Build history of the part. All positions in model axes, mm. Round coordinates to 2 decimals unless told otherwise and drop trailing zeros. Loops run counter-clockwise (first coordinate to the right, second up) from the corner with the lowest first, then second, coordinate; pieces in that order, holes last. Notation, with made-up numbers: M 74.25,68 L 125.25,68 A19 cw 125.25,100 Z; hole C 53.5,61.25 d1. An arc over 180 degrees is marked long. Use one line per item in the form item = value. Start each with the question number.
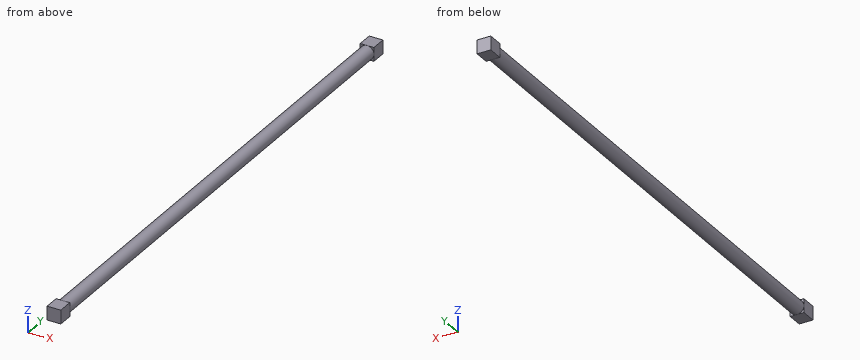
```python
from build123d import *

# Parameters (mm, degrees)
F0_R     = 5.715
F1_DEPTH = 457.2
F2_W     = 11.43
F2_H     = 11.43
F3_DEPTH = 12.7
F4_W     = 11.43
F4_H     = 11.43
F5_DEPTH = 12.7


with BuildPart() as f1:
    # F0 (on Front) → F1 (new body)
    with BuildSketch(Plane.XZ):
        Circle(F0_R)
    extrude(amount=F1_DEPTH)

    # F2 (on face) → F3 (join)
    with BuildSketch(Plane(origin=(0, 0, 0), x_dir=(-1, 0, 0), z_dir=(0, 1, 0))):
        Rectangle(F2_W, F2_H)
    extrude(amount=-F3_DEPTH)

    # F4 (on face) → F5 (join)
    with BuildSketch(Plane.XZ.offset(457.2)):
        Rectangle(F4_W, F4_H)
    extrude(amount=-F5_DEPTH)


solid = f1.part
```
Q1. Wall check: probe 1 along Y at (x, z) = (5.25, -5); probe 2 along Z at (x, y) = (0.25, -436.5); probe 3 along Z at (x, y) = (1, -319). Give the ranges that are in metal, low to high.
Q2. Saw through at C-C (y = -225). Give the cut face in (x, z) (3 decimals).
Q3. Saw through at B-B (z = 1.75). Give the cut face in (x, y) (3 decimals).
Q4. Drop flat-ended pins along their axis: P1, Ø4.5, axis at x = -3.5, z = 3.5, coming from the +Y side; P2, Ø2, axis at y = -92, z = -2, coming from the -X side; P3, Ø2, axis at x = -4, y = -174.5, coming from the +Z side. Give the stop position or say it passes through.
Q5. Saw through at A-A (x = -2.5). Give the cut face in (y, z) (3 decimals), and give its area (3 significant figures).
Filled in:
q1.probe_1 = -457.2 to -444.5, -12.7 to 0
q1.probe_2 = -5.71 to 5.71
q1.probe_3 = -5.63 to 5.63
q2.outline = C 0,0 d11.43
q3.outline = M -5.715,-457.2 L 5.715,-457.2 L 5.715,-444.5 L 5.44,-444.5 L 5.44,-12.7 L 5.715,-12.7 L 5.715,0 L -5.715,0 L -5.715,-12.7 L -5.44,-12.7 L -5.44,-444.5 L -5.715,-444.5 Z
q4.P1 = 0
q4.P2 = -5.63
q4.P3 = 4.86
q5.outline = M -457.2,-5.715 L -444.5,-5.715 L -444.5,-5.139 L -12.7,-5.139 L -12.7,-5.715 L 0,-5.715 L 0,5.715 L -12.7,5.715 L -12.7,5.139 L -444.5,5.139 L -444.5,5.715 L -457.2,5.715 Z
q5.area = 4,730 mm²
